Read the model definition and answer for the solid it produces. Units are mm, in the model's axes. Coordinates: 2 decimals unless noted, no trailing zeros. Order: outer loops, then holes, each group sorted by start corner. A loop starts at its lowest first (then second) coordinate and runs counter-clockwise, first axis right, second up. Notation, with made-up numbers: M -29,11.5 L 7,11.5 A9 ccw 7,22.5 Z; hole C 64.5,19 d7. An arc over 180 degrees is marked long. Write each question's results on one line, items separated by ' | '.
```python
from build123d import *
from OCP.BRepFilletAPI import BRepFilletAPI_MakeChamfer

# Parameters (mm, degrees)
BOSS_EXTRUDE1_DEPTH      = 2.38125
BOSS_EXTRUDE1_DEPTH_BACK = 2.38125
CHAMFER1_SIZE            = 1.5875
CHAMFER1_SIZE2           = 6.35
CHAMFER3_SIZE            = 6.35
CHAMFER3_SIZE2           = 1.5875


with BuildPart() as part:
    # Sketch1 → Boss-Extrude1 (new, two sides: drawn at the far end of the back side and taken through both)
    with BuildSketch(Plane(origin=(0, 0, 0), x_dir=(1, 0, 0), z_dir=(0, 1, 0)).offset(-BOSS_EXTRUDE1_DEPTH_BACK)):
        Polygon((0, 0), (0, 25.4), (76.2, 127), (152.4, 127), (203.2, 25.4), (203.2, 0), align=None)
    extrude(amount=BOSS_EXTRUDE1_DEPTH + BOSS_EXTRUDE1_DEPTH_BACK)

    # Chamfer1: one chamfer whose edges measure the first distance from different faces: ONE call of the kernel's chamfer builder (chamfer() names one face for all edges)
    chamfer1_edges_1 = [part.edges().sort_by_distance(p)[0] for p in [
        (177.8, 2.38125, -76.2),
        (177.8, -2.38125, -76.2),
    ]]
    chamfer1_side_1 = [part.faces().sort_by_distance(p)[0] for p in [
        (177.8, 0, -76.2),
    ]]
    chamfer1_edges_2 = [part.edges().sort_by_distance(p)[0] for p in [
        (38.1, -2.38125, -76.2),
    ]]
    chamfer1_side_2 = [part.faces().sort_by_distance(p)[0] for p in [
        (38.1, 0, -76.2),
    ]]
    chamfer1 = BRepFilletAPI_MakeChamfer(part.part.solid().wrapped)
    for e in chamfer1_edges_1:
        chamfer1.Add(CHAMFER1_SIZE, CHAMFER1_SIZE2, e.wrapped, chamfer1_side_1[0].wrapped)  # the first distance lies on this face
    for e in chamfer1_edges_2:
        chamfer1.Add(CHAMFER1_SIZE, CHAMFER1_SIZE2, e.wrapped, chamfer1_side_2[0].wrapped)  # the first distance lies on this face
    add(Compound.cast(chamfer1.Shape()), mode=Mode.REPLACE)

    # Chamfer3
    chamfer3_edges = [part.edges().sort_by_distance(p)[0] for p in [
        (38.1, 2.38125, -76.2),
    ]]
    chamfer3_side = [part.faces().sort_by_distance(p)[0] for p in [
        (102.626088035, 2.38125, -52.835240535),
    ]]
    chamfer(chamfer3_edges, length=CHAMFER3_SIZE, length2=CHAMFER3_SIZE2, reference=chamfer3_side[0])


solid = part.part
```
(1) The part is cut by section C-C, the plane z = -39. Write down the section's boundary in (x, y).
Conclusion:
outline: M 10.2,-0.79 L 18.14,-2.38 L 189.3,-2.38 L 196.4,-0.79 L 196.4,0.79 L 189.3,2.38 L 18.14,2.38 L 10.2,0.79 Z
(2) The part is cut by section D-D, the plane x = 27. Write down the section's boundary in (y, z), then the cut area to 3 significant figures.
Conclusion:
outline: M -2.38,-50.82 L -0.79,-61.4 L 0.79,-61.4 L 2.38,-50.82 L 2.38,0 L -2.38,0 Z | area: 276 mm²
(3) Given pin 1 (2 mm diameter, centred on y = 1.5, z = -68.5, fed in from +X); pin 2 (1 mm diameter, centred on x = 131, y = 1, fed in from +Z), each flat-ended and moving along its own axis, determine where each tip first touches the part or whether it passes through.
Conclusion:
pin 1: x = 182 | pin 2: z = 0
(4) The part is cut by section A-A, the plane z = -96. Write down the section's boundary in (x, y).
Conclusion:
outline: M 52.95,-0.79 L 60.89,-2.38 L 160.8,-2.38 L 167.9,-0.79 L 167.9,0.79 L 160.8,2.38 L 60.89,2.38 L 52.95,0.79 Z
(5) Straight lines are drawn through the part: line 1 (Y direction, x = 19, z = -50.5); line 2 (Z direction, x = 64.5, y = -0.1); line 3 (Z direction, x = 183, y = -0.1). For each, find the intervals that lie inside material, in ascending order.
Conclusion:
line 1: -0.83 to 0.83 | line 2: -111.4 to 0 | line 3: -65.8 to 0
(6) The part is cut by section B-B, the plane x = 52.5. Write down the section's boundary in (y, z), then the cut area to 3 significant figures.
Conclusion:
outline: M -2.38,-84.82 L -0.79,-95.4 L 0.79,-95.4 L 2.38,-84.82 L 2.38,0 L -2.38,0 Z | area: 438 mm²
